The model under review builds one solid part; all positions refer to its coordinate system, in mm. A direction names the side the tool comes from. Coordinates: 2 decimals unless noted, no trailing zeros. Write each loop counter-clockwise with the first axis right and the second up, starting at its lowest first coordinate (ties: lowest second). Pieces come first, ordered by that corner, then holes. Notation, with made-up numbers: (-30, 45.25) -> (29, 45.25) arc R15 cw to (29, 58.25) -> close; hole circle Ø3 at (-24.75, -35.5). An arc over 180 degrees is marked (long way). Put each result on its own line as item: value. Start each with the question number.
Autodesk Inventor part; units mm, degrees
ref_plane "YZ Plane" through (0, 0, 0) normal (1, 0, 0) x (0, 1, 0)
ref_plane "XZ Plane" through (0, 0, 0) normal (0, 1, 0) x (-1, 0, 0)
ref_plane "XY Plane" through (0, 0, 0) normal (0, 0, 1) x (1, 0, 0)
sketch "Sketch1" plane through (0, 0, 0) normal (0, 1, 0) x (-1, 0, 0)
  line L0 (37, 37) -> (-37, 37)
  line L1 (-37, 37) -> (-37, -37)
  line L2 (-37, -37) -> (37, -37)
  line L3 (37, -37) -> (37, 37)
  point P0 (0, 0)
  dimension "d0" = 74
  dimension "d1" = 74
extrude "Extrusion1" add sketch "Sketch1" along normal blind 6
fillet "Fillet1" radius 5 4 edges at (-37, 3, 37) (37, 3, 37) (37, 3, -37) (-37, 3, -37)
fillet "Fillet2" radius 2 8 edges at (35.5355, 0, 35.5355) (37, 0, 0) (35.5355, 0, -35.5355) (0, 0, -37) (-35.5355, 0, -35.5355) (-37, 0, 0) (-35.5355, 0, 35.5355) (0, 0, 37)
sketch "Sketch6" plane through (0, 6, 0) normal (0, 1, 0) x (1, 0, 0)
  circle A0 centre (0, 0) radius 3
  circle A1 centre (6.2, 23.4) radius 2
  circle A2 centre (-8.8, 23.4) radius 2
  line L0 (-1.3, 4) -> (-13.3, 4)
  line L1 (-13.3, 4) -> (-13.3, 19)
  line L2 (-13.3, 19) -> (-1.3, 19)
  line L3 (-1.3, 19) -> (-1.3, 4)
  line L4 (17.5, -5) -> (-17.5, -5)
  line L5 (-17.5, -5) -> (-17.5, -18)
  line L6 (-17.5, -18) -> (17.5, -18)
  line L7 (17.5, -18) -> (17.5, -5)
  dimension "d29" = 6
  dimension "d30" = 4
  dimension "d31" = 4
  dimension "d32" = 12
  dimension "d33" = 15
  dimension "d34" = 35
  dimension "d35" = 13
extrude "Extrusion6" cut sketch "Sketch6" against normal blind 10
sketch "Sketch7" plane through (0, 6, 0) normal (0, 1, 0) x (1, 0, 0)
  circle A0 centre (0, -32) radius 2
  point P0 (0, 0)
  dimension "d38" = 4
extrude "Extrusion7" cut sketch "Sketch7" against normal blind 10
pattern_circular "Circular Pattern1" count 4 over 360 about axis through (0, -10, 0) along (0, 1, 0) of "Extrusion7"
properties part number "g2ExtruMountPlate"
1. The part is to be moulded in two halves that separate along Z. For faces 3 (the cylindrical face through (-34, 3, 0)), 4 (the flat face through (-13.3, 3, -11)), 5 (the flat face through (-37, 4, 0)), 6 (the cylindrical face through (-36, 4, 35)), say which applies: released by +Z, released by -Z, zero draft, split by the parting line, or undercut.
2. Tool access review of faces 1 (the flat face through (0, 0, -7)), 2 (the flat face through (-7, 3, -19)): name each direction out of +Z, -Z, +X, -X, +Y, -Y from which nothing blocks a thin tool from reaching the whole face with its end or side.
3. Insertion check: P1, Ø2.5, axis at x = 32, z = 0, coming from the -Y side. The pin has a flat end and moves straight along its axis. Give the tip position at first contact, or say it passes through.
4. Consider section C-C on z = -23.4. State the section outline as (x, y) points.
5. Consider section A-A on z = 0. State the section outline as (x, y) points.
6. Wall thickness on line 1 (X direction, y = 2.3, z = -23.4); line 2 (Z direction, x = -9, y = 3); line 3 (X direction, y = 4.8, z = 0): over which ranges is each line inside the solid? List them lowest first. Write a range as from..to.
7. Consider section B-B on x = -8.8. State the section outline as (y, z) points.
8. Consider section D-D on y = 5.1. State how many separate pieces and enclosed holes the cut face has, then the cut area to 3 significant figures.
Output values:
1. face 3: undercut
1. face 4: undercut
1. face 5: zero draft
1. face 6: released by +Z
2. face 1: +Z, -Z, +X, -X, -Y
2. face 2: +Y, -Y
3. P1: passes through
4. outline: (-37, 2) arc R2 ccw to (-35, 0) -> (-10.8, 0) -> (-10.8, 6) -> (-37, 6) -> close; (-6.8, 0) -> (4.2, 0) -> (4.2, 6) -> (-6.8, 6) -> close; (8.2, 0) -> (35, 0) arc R2 ccw to (37, 2) -> (37, 6) -> (8.2, 6) -> close
5. outline: (-37, 2) arc R2 ccw to (-35, 0) -> (-34, 0) -> (-34, 6) -> (-37, 6) -> close; (-30, 0) -> (-3, 0) -> (-3, 6) -> (-30, 6) -> close; (3, 0) -> (30, 0) -> (30, 6) -> (3, 6) -> close; (34, 0) -> (35, 0) arc R2 ccw to (37, 2) -> (37, 6) -> (34, 6) -> close
6. line 1: x = -37..-10.8, -6.8..4.2, 8.2..37
6. line 2: z = -37..-25.39, -21.41..-19, -4..5, 18..37
6. line 3: x = -37..-34, -30..-3, 3..30, 34..37
7. outline: (0, -35) arc R2 ccw to (2, -37) -> (6, -37) -> (6, -25.4) -> (0, -25.4) -> close; (0, -21.4) -> (6, -21.4) -> (6, -19) -> (0, -19) -> close; (0, -4) -> (6, -4) -> (6, 5) -> (0, 5) -> close; (0, 18) -> (6, 18) -> (6, 37) -> (2, 37) arc R2 ccw to (0, 35) -> close
8. separate pieces: 1
8. enclosed holes: 9
8. area: 4,720 mm^2
